Can you work these out from the drawing? Everything is in mm from the part's minimum corner. A direction names the side the tool comes from. Give positions to 0.01 mm unless a question says otherwise; leave off trailing zeros. Loops run counter-clockwise (first coordinate to the right, second up) from the corner with the lowest first, then second, coordinate; pieces in that order, holes last. Notation, with made-up numbers: (-37.5, 22.5) - (8.5, 22.5) arc R25 cw to (8.5, 59.5) - close; hole circle Ø1 at (4, -25.5). An arc over 180 degrees is marked (long way). One line per item, written item: value. Start each with the question number.
Q1. I want a section at B-B (y = 10.75). Please give me the cut outline in (x, z) (1 decimal).
Q2. If I drill on line 1 (X direction, y = 2.15, z = 107.95); line 2 (X direction, y = 15.25, z = 88); line 3 (Z direction, x = 97, y = 2.5) (1 decimal), over which ranges is the centre line in solid material (lowest first)? Write a range as from..to.
Q3. I want a section at A-A (z = 95.25). Please give me the cut outline in (x, y) (1 decimal).
Q4. For the marked faces 1 and 2, which set-ups out of +Z, -Z, +X, -X, +Y, -Y let a thin tool reach every point of the face, with its end or its side?
Q5. If we mould it in two halves opening along X, with no side actions, what happens to the marked faces 3, 4 and 5? For each: released by +X, released by -X, zero draft, split by the parting line, or undercut.
Q6. I'm going to push flat-ended pins straight in: P1, Ø10, axis at x = 76, z = 58.5, coming from the -Y side; P2, Ø10, axis at x = 81, y = 17, coming from the +Z side; P3, Ø3, axis at x = 100, y = 10.5, coming from the +Z side (3 decimals); P4, Ø4, axis at x = 98.425, z = 95.25, coming from the +Y side (3 decimals). Where does each tip first touch, or does it pass through?
Q7. I want a section at C-C (x = 45). Please give me the cut outline in (y, z) (1 decimal).
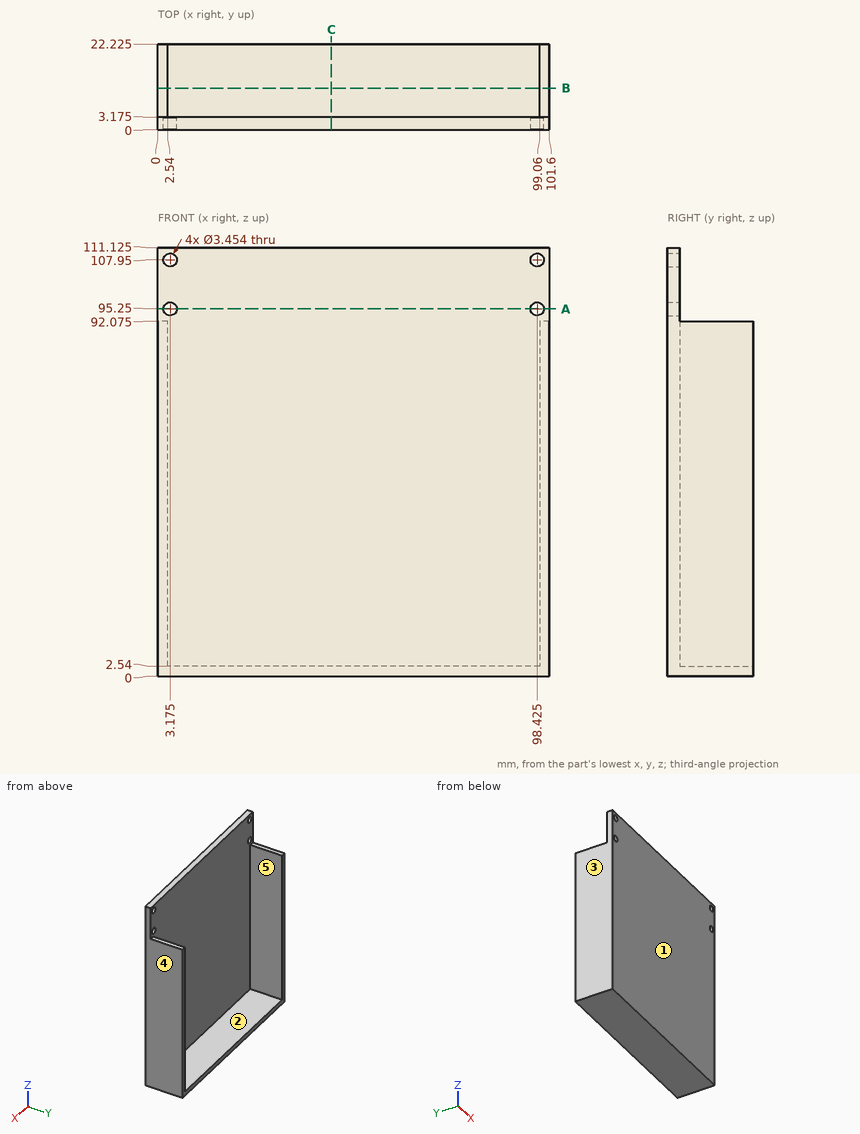
Worked answers:
1. outline: (0, 0) - (101.6, 0) - (101.6, 92.1) - (99.1, 92.1) - (99.1, 2.5) - (2.5, 2.5) - (2.5, 92.1) - (0, 92.1) - close
2. line 1: x = 0..1.45, 4.9..96.7, 100.15..101.6
2. line 2: x = 0..2.54, 99.06..101.6
2. line 3: z = 0..94.3, 96.2..107, 108.9..111.1
3. outline: (0, 0) - (1.4, 0) - (1.4, 3.2) - (0, 3.2) - close; (4.9, 0) - (96.7, 0) - (96.7, 3.2) - (4.9, 3.2) - close; (100.2, 0) - (101.6, 0) - (101.6, 3.2) - (100.2, 3.2) - close
4. face 1: +Z, -Z, +X, -X, -Y
4. face 2: +Z, +Y
5. face 3: released by -X
5. face 4: released by +X
5. face 5: undercut
6. P1: stops at y = 0
6. P2: stops at z = 2.54
6. P3: stops at z = 92.075
6. P4: stops at y = 3.175
7. outline: (0, 0) - (22.2, 0) - (22.2, 2.5) - (3.2, 2.5) - (3.2, 111.1) - (0, 111.1) - close
